Read the model definition and answer for the solid it produces. Units are mm, in the model's axes. A direction names the side the tool comes from. Give positions to 0.01 mm unless a question says otherwise; leave off trailing zeros. Loops run counter-clockwise (first coordinate to the right, second up) from the corner with the lowest first, then second, coordinate; pieces in that order, holes last.
(1) Find section A-A, the plane x = 0. Write down the section's boundary in (y, z), then the cut area to 3 significant figures.
(2) Straight lines are drawn through the part: probe 1 along Z at (x, y) = (-21, -7); probe 2 along Y at (x, z) = (24.5, 22); probe 3 along Y at (x, z) = (0, -2). For each, find the intervals that lie inside material, in ascending order.
(3) Which of the six approach directions +Z, -Z, +X, -X, +Y, -Y give full straight-line access (tool end or side, diameter ignored) to faces 4 (the face through (17, 16, -3)), 5 (the face through (-2.17, -0.81, -1.61)), 6 (the face through (23, 16.25, 12)), 7 (the face through (-17, 15, -3))?
(4) Find section C-C, the plane y = 13. Write down the section's boundary in (x, z).
(5) Determine the mould class of faces 1 (the face through (-2.17, -0.81, 22.54)), 2 (the face through (30, -1, 12)), 3 (the face through (-29.26, 15.49, 12.33)) for opening direction X: pulls with the +X half, pulls with the -X half, needs draft (parallel to the pull), parting line crosses it, or undercut.
(6) Each of these flat-tipped pins is pushed along its axis until it touches: P1, Ø3.5, axis at x = -21, z = 10, coming from the +Y side; P2, Ø16, axis at x = 0, y = 8.95, coming from the +Z side; P3, Ø11, axis at x = 0, y = 8.95, coming from the +Z side; P4, Ø2, axis at x = -13, z = -4.5, coming from the -Y side. Where does it stop, or does it pass through?
(7) Find section B-B, the plane z = 3.5. Write down the section's boundary in (x, y).
(8) Find section D-D, the plane x = 13. Write down the section's boundary in (y, z), then the cut area to 3 significant figures.
```python
from build123d import *

# Parameters (mm, degrees)
CROQUIS1_W              = 60
CROQUIS1_H              = 32.5
SALIENTE_EXTRUIR1_DEPTH = 25
SALIENTE_EXTRUIR2_DEPTH = 34
CROQUIS3_R              = 6
CORTAR_EXTRUIR1_DEPTH   = 35
CHAFL_N1_SIZE           = 1.5
CHAFL_N2_SIZE           = 1.5
CHAFL_N3_SIZE           = 1.5
CROQUIS5_R              = 10
CORTAR_EXTRUIR2_DEPTH   = 15
CROQUIS6_R              = 10
CORTAR_EXTRUIR3_DEPTH   = 5


with BuildPart() as part:
    # Croquis1 → Saliente-Extruir1 (new body)
    with BuildSketch(Plane.XY):
        Rectangle(CROQUIS1_W, CROQUIS1_H)
    extrude(amount=SALIENTE_EXTRUIR1_DEPTH)

    # Croquis2 → Saliente-Extruir2 (add)
    with BuildSketch(Plane(origin=(0, 0, 25), x_dir=(-1, 0, 0), z_dir=(0, 0, -1))):
        Polygon((-17, 16.25), (-17, 26.75), (17, 26.75), (17, 16.25), (17, -9.25), (-17, -9.25), align=None)
    extrude(amount=SALIENTE_EXTRUIR2_DEPTH)

    # Croquis3 → Cortar-Extruir1 (cut, through all)
    with BuildSketch(Plane(origin=(0, 0, 25), x_dir=(-1, 0, 0), z_dir=(0, 0, -1))):
        with Locations((0, 8.95)):
            Circle(CROQUIS3_R)
    extrude(amount=CORTAR_EXTRUIR1_DEPTH, mode=Mode.SUBTRACT)

    # Chaflán1
    chafl_n1_edges = [part.edges().sort_by_distance(p)[0] for p in [
        (17, 26.75, 8),
    ]]
    chamfer(chafl_n1_edges, length=CHAFL_N1_SIZE)

    # Chaflán2
    chafl_n2_edges = [part.edges().sort_by_distance(p)[0] for p in [
        (-17, 26.75, 8),
    ]]
    chamfer(chafl_n2_edges, length=CHAFL_N2_SIZE)

    # Chaflán3
    chafl_n3_edges = [part.edges().sort_by_distance(p)[0] for p in [
        (-30, 16.25, 12.5),
        (30, 16.25, 12.5),
    ]]
    chamfer(chafl_n3_edges, length=CHAFL_N3_SIZE)

    # Croquis5 → Cortar-Extruir2 (cut)
    with BuildSketch(Plane.XY.offset(-9)):
        with Locations((0, 8.95)):
            Circle(CROQUIS5_R)
    extrude(amount=CORTAR_EXTRUIR2_DEPTH, mode=Mode.SUBTRACT)

    # Croquis6 → Cortar-Extruir3 (cut)
    with BuildSketch(Plane.XY.offset(25)):
        with Locations((0, 8.95)):
            Circle(CROQUIS6_R)
    extrude(amount=-CORTAR_EXTRUIR3_DEPTH, mode=Mode.SUBTRACT)


solid = part.part
```
Entries:
1. outline: (-16.25, 0) - (-9.25, 0) - (-9.25, -9) - (-1.05, -9) - (-1.05, 6) - (2.95, 6) - (2.95, 20) - (-1.05, 20) - (-1.05, 25) - (-16.25, 25) - close; (14.95, 6) - (18.95, 6) - (18.95, -9) - (26.75, -9) - (26.75, 25) - (18.95, 25) - (18.95, 20) - (14.95, 20) - close
1. area: 831 mm2
2. probe 1: z = 0 to 25
2. probe 2: y = -16.25 to 16.25
2. probe 3: y = -9.25 to -1.05, 18.95 to 26.75
3. face 4: -Z, +X, +Y
3. face 5: -Z
3. face 6: +Z, -Z, +X, +Y
3. face 7: -Z, -X, +Y
4. outline: (-30, 0) - (-17, 0) - (-17, -9) - (-9.14, -9) - (-9.14, 6) - (-4.43, 6) - (-4.43, 20) - (-9.14, 20) - (-9.14, 25) - (-30, 25) - close; (4.43, 6) - (9.14, 6) - (9.14, -9) - (17, -9) - (17, 0) - (30, 0) - (30, 25) - (9.14, 25) - (9.14, 20) - (4.43, 20) - close
5. face 1: undercut
5. face 2: pulls with the +X half
5. face 3: pulls with the -X half
6. P1: stops at y = 16.25
6. P2: stops at z = 20
6. P3: passes through
6. P4: stops at y = -9.25
7. outline: (-30, -16.25) - (30, -16.25) - (30, 14.75) - (28.5, 16.25) - (17, 16.25) - (17, 25.25) - (15.5, 26.75) - (-15.5, 26.75) - (-17, 25.25) - (-17, 16.25) - (-28.5, 16.25) - (-30, 14.75) - close; hole circle Ø20 at (0, 8.95)
8. outline: (-16.25, 0) - (-9.25, 0) - (-9.25, -9) - (26.75, -9) - (26.75, 25) - (-16.25, 25) - close
8. area: 1,400 mm2
